```python
from build123d import *

# Parameters (mm, degrees)
F1_DEPTH = 3


with BuildPart() as f1:
    # F0 (on Top) → F1 (new body)
    with BuildSketch(Plane.XY):
        with BuildLine():
            Line((-20, -25), (20, -25))
            ThreePointArc((20, -25), (23.535534, -23.535534), (25, -20))
            Line((25, -20), (25, 20))
            ThreePointArc((25, 20), (23.535534, 23.535534), (20, 25))
            Line((20, 25), (15, 25))
            ThreePointArc((15, 25), (11.464466, 26.464466), (10, 30))
            Line((10, 30), (10, 37))
            ThreePointArc((10, 37), (0, 47), (-10, 37))
            Line((-10, 37), (-10, 30))
            ThreePointArc((-10, 30), (-11.464466, 26.464466), (-15, 25))
            Line((-15, 25), (-20, 25))
            ThreePointArc((-20, 25), (-23.535534, 23.535534), (-25, 20))
            Line((-25, 20), (-25, -20))
            ThreePointArc((-25, -20), (-23.535534, -23.535534), (-20, -25))
        make_face()
        with BuildLine():
            ThreePointArc((0, 30), (-4.949747, 41.949747), (7, 37))
            ThreePointArc((7, 37), (4.949747, 32.050253), (0, 30))
        make_face(mode=Mode.SUBTRACT)
    extrude(amount=F1_DEPTH)


solid = f1.part
```
Design review of the part built by this model. Coordinates are the model's own, in mm. A direction names the side the tool comes from. Coordinates: 2 decimals unless noted, no trailing zeros. Order: outer loops, then holes, each group sorted by start corner. A loop starts at its lowest first (then second) coordinate and runs counter-clockwise, first axis right, second up. Notation, with made-up numbers: (79, 66) - (88, 66) arc R19 cw to (88, 83) - close; hole circle Ø7 at (-11.5, -28.75). An arc over 180 degrees is marked (long way). Answer in a Markdown table with one row per item.
(1) Clearance check with flat-ended pins moving along their axes: pin 1 (1 mm diameter, centred on x = 5, z = 1.5, fed in from +Y); pin 2 (1.5 mm diameter, centred on y = 32.5, z = 2, fed in from +X); pin 3 (11 mm diameter, centred on x = 0, y = 37, fed in from +Z); pin 4 (1.5 mm diameter, centred on x = 18, z = 2, fed in from +Y). State where each tip first meets the part, or that it passes through.
Checked values:
| item | result |
|---|---|
| pin 1 | y = 45.93 |
| pin 2 | x = 10 |
| pin 3 | through |
| pin 4 | y = 25 |
(2) Consider section A-A on z = 0.5. State the section outline as (x, y) points.
Checked values:
| item | result |
|---|---|
| outline | (-25, -20) arc R5 ccw to (-20, -25) - (20, -25) arc R5 ccw to (25, -20) - (25, 20) arc R5 ccw to (20, 25) - (15, 25) arc R5 cw to (10, 30) - (10, 37) arc R10 ccw to (-10, 37) - (-10, 30) arc R5 cw to (-15, 25) - (-20, 25) arc R5 ccw to (-25, 20) - close; hole (0, 30) arc R7 ccw to (7, 37) arc R7 ccw (long way) to start |
(3) Wall thickness on line 1 along X through (y, z) = (37, 1.1); line 2 along Y through (x, z) = (0, 1.45); line 3 along Y through (x, z) = (20, 0.45): over which ranges is each line inside the solid? List them lowest first. Write a range as from..to.
Checked values:
| item | result |
|---|---|
| line 1 | -10..-7, 7..10 |
| line 2 | -25..30, 44..47 |
| line 3 | -25..25 |
(4) For faces 1 (the cylindrical face through (0, 47, 1)), 2 (the flat face through (-10, 34, 1)), 3 (the flat face through (10, 33, 1)), list the 3-axis set-ups (+Z, -Z, +X, -X, +Y, -Y) from which the entire face can be reached by the end or side of a thin tool; tool diameter is ignored.
Checked values:
| item | result |
|---|---|
| face 1 | +Z, -Z, +Y |
| face 2 | +Z, -Z, -X, +Y |
| face 3 | +Z, -Z, +X, +Y |
(5) Consider section B-B on x = -21. State the section outline as (y, z) points.
Checked values:
| item | result |
|---|---|
| outline | (-24.9, 0) - (24.9, 0) - (24.9, 3) - (-24.9, 3) - close |
